Autodesk Inventor part; units mm, degrees
ref_plane "YZ Plane" through (0, 0, 0) normal (1, 0, 0) x (0, 1, 0)
ref_plane "XZ Plane" through (0, 0, 0) normal (0, 1, 0) x (-1, 0, 0)
ref_plane "XY Plane" through (0, 0, 0) normal (0, 0, 1) x (1, 0, 0)
sketch "Sketch1" plane through (0, 0, 0) normal (0, 0, 1) x (1, 0, 0)
  line L0 (0, 0) -> (0, 54.375)
  line L1 (0, 54.375) -> (192, 54.375)
  line L2 (0, 0) -> (772.3927, 0)
  line L3 (253.9225, 18.624) -> (253.9225, 0) construction
  line L4 (192, 54.375) -> (253.9225, 18.624)
  line L5 (253.9225, 18.624) -> (256.9225, 18.624)
  line L6 (256.9225, 18.624) -> (325.3908, 36.97)
  line L7 (325.3908, 36.97) -> (325.3908, 0)
  line L8 (192, 54.375) -> (192, 0)
  line L9 (0, 54.375) -> (0, 69.375)
  line L10 (0, 69.375) -> (20, 69.375)
  line L11 (20, 69.375) -> (20, 58.375)
  line L12 (192, 54.375) -> (192, 74.375)
  line L13 (20, 58.375) -> (172, 58.375)
  line L14 (172, 58.375) -> (192, 58.375)
  dimension "d9" = 54.375
  dimension "d10" = 192
  dimension "d12" = 18.624
  dimension "d13" = 150
  dimension "d15" = 3
  dimension "d16" = 15
  dimension "d17" = 36.97
  dimension "d18" = 518.4701
  dimension "d19" = 15
  dimension "d20" = 20
  dimension "d21" = 11
revolve "Revolution2" add sketch "Sketch1" angle 360 about axis through (0, 0, 0) along (1, 0, 0) contours L9 L10 L11 L13 L14 L12 L1
properties part number "combustion chamber" material "Stainless Steel, Austenitic"
Part model, mm, in its own coordinate system. A direction names the side the tool comes from. Coordinates: 2 decimals unless noted, no trailing zeros. Write each loop counter-clockwise with the first axis right and the second up, starting at its lowest first coordinate (ties: lowest second). Pieces come first, ordered by that corner, then holes.
Item 1: Mould opens along Z. For faces 3 (the face through (0, -41, -36)), 4 (the face through (97.34, -11.79, -53.08)), 5 (the face through (10.14, -9.031, 68.785)) say: released by +Z, released by -Z, zero draft, split by the parting line, or undercut.
Item 2: Pin check, flat tips, straight feed: pin 1 (5 mm diameter, centred on x = 170, y = -15.5, fed in from -Z); pin 2 (4 mm diameter, centred on y = -36, z = 53, fed in from +X); pin 3 (2 mm diameter, centred on x = 39.5, y = -12.5, fed in from +Z). Stop position of each tip, or through.
Item 3: Which spindle directions (+Z, -Z, +X, -X, +Y, -Y) get a long thin tool onto all of the face, cutting with end or side? Do faces 1 (the face through (192, -48, 26)), 2 (the face through (107.204, -12.655, -56.987)). Say none if no direction does.
Item 4: Slice it at C-C (x = 48.5). Write the cut outline in (y, z) (3 decimals).
Item 5: Slice it at A-A (y = 0). Write the cut outline in (x, z) (3 decimals), and give its area (3 significant figures).
Item 6: Probe line 1 (Z direction, x = 145.5, y = 0) (3 decimals); line 2 (Y direction, x = 114.5, z = 4); line 3 (Y direction, x = 72, z = 5). List the from-to ranges inside material, lowest first.
Results found:
1. face 3: zero draft
1. face 4: undercut
1. face 5: split by the parting line
2. pin 1: stops at z = -56.91
2. pin 2: stops at x = 20
2. pin 3: stops at z = 57.23
3. face 1: +Z, -Z, +X, +Y, -Y
3. face 2: +X
4. outline: circle Ø116.75 at (0, 0); hole circle Ø108.75 at (0, 0)
5. outline: (0, -69.375) - (20, -69.375) - (20, -58.375) - (192, -58.375) - (192, -54.375) - (0, -54.375) - close; (0, 54.375) - (192, 54.375) - (192, 58.375) - (20, 58.375) - (20, 69.375) - (0, 69.375) - close
5. area: 1,980 mm2
6. line 1: z = -58.375 to -54.375, 54.375 to 58.375
6. line 2: y = -58.24 to -54.23, 54.23 to 58.24
6. line 3: y = -58.16 to -54.14, 54.14 to 58.16
